The figure shows three views and two pictorial views of one solid part (mm, origin at its lowest corner). Answer the questions. Coordinates: 2 decimals unless noted, no trailing zeros. Order: outer loops, then holes, each group sorted by start corner. A loop starts at its lowest first (then second) coordinate and runs counter-clockwise, first axis right, second up. Notation, with made-up numbers: (86, -40) - (119, -40) arc R13 cw to (119, -33) - close; hole circle Ø7 at (15, -9.5). An arc over 180 degrees is marked (long way). Use one line per item in the form item = value.
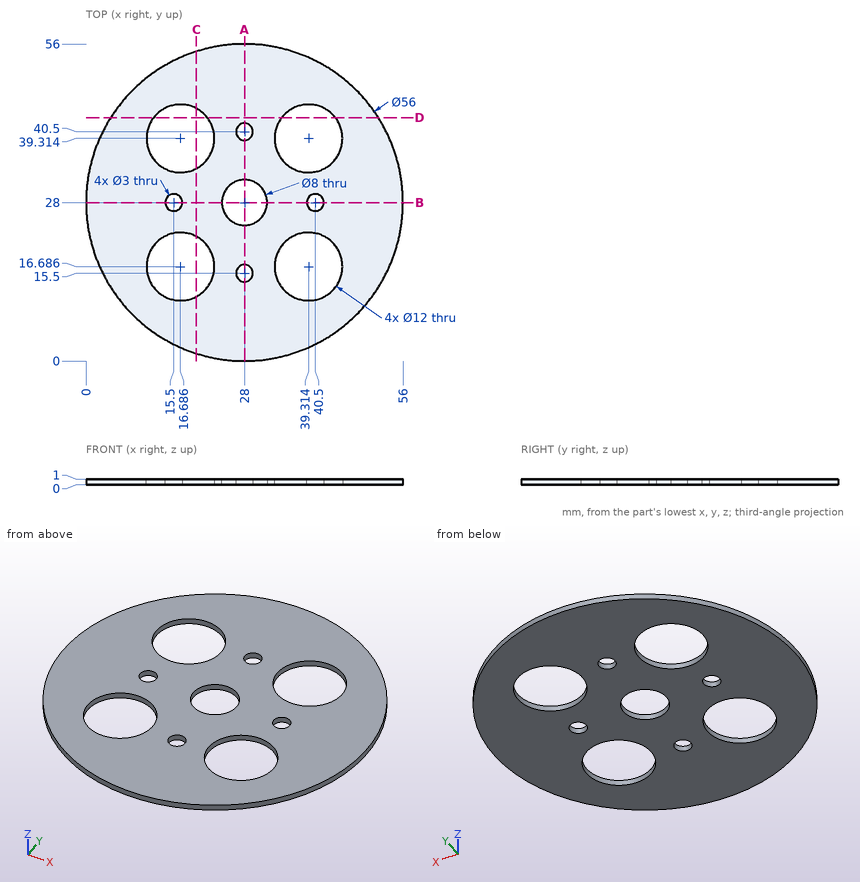
(1) Straight lines are drawn through the part: L1, parallel to Y at x = 28, z = 0.7; L2, parallel to Y at x = 13.5, z = 0.25. For each, find the intervals that lie inside material, in ascending order.
Answer list:
L1 = 0 to 14, 17 to 24, 32 to 39, 42 to 56
L2 = 4.05 to 11.6, 21.77 to 34.23, 44.4 to 51.95
(2) Given pin 1 Ø2.5 at (x, y) = (28, 40.5) entering from +Z, flat-ended and moving along its own axis, determine where the tip first touches the part or whether it passes through.
Answer list:
pin_1 = through
(3) Section A-A, the plane x = 28 is taken. Write down the section's boundary in (y, z).
Answer list:
outline = (0, 0) - (14, 0) - (14, 1) - (0, 1) - close; (17, 0) - (24, 0) - (24, 1) - (17, 1) - close; (32, 0) - (39, 0) - (39, 1) - (32, 1) - close; (42, 0) - (56, 0) - (56, 1) - (42, 1) - close
(4) Section D-D, the plane y = 43 is taken. Write down the section's boundary in (x, z).
Answer list:
outline = (4.36, 0) - (11.95, 0) - (11.95, 1) - (4.36, 1) - close; (21.42, 0) - (34.58, 0) - (34.58, 1) - (21.42, 1) - close; (44.05, 0) - (51.64, 0) - (51.64, 1) - (44.05, 1) - close
(5) Section C-C, the plane x = 19.5 is taken. Write down the section's boundary in (y, z).
Answer list:
outline = (1.32, 0) - (11.39, 0) - (11.39, 1) - (1.32, 1) - close; (21.99, 0) - (34.01, 0) - (34.01, 1) - (21.99, 1) - close; (44.61, 0) - (54.68, 0) - (54.68, 1) - (44.61, 1) - close
